The model under review builds one solid part; all positions refer to its coordinate system, in mm. A direction names the side the tool comes from. Coordinates: 2 decimals unless noted, no trailing zeros. Loops run counter-clockwise (first coordinate to the right, second up) from the corner with the lowest first, then second, coordinate; pieces in that order, holes last. Notation, with made-up numbers: (44, 87.25) - (57, 87.25) arc R35 cw to (57, 121.25) - close; hole circle Ø1 at (66.25, 66). An arc over 180 degrees is marked (long way). Answer in a Markdown table with one row per item. Add a question column.
(1) For P1, Ø5, axis at x = -135.5, z = 30, coming from the -Y side; P2, Ø4, axis at y = 152, z = 42.5, coming from the +X side; P3, Ø1, axis at x = -95, z = 32, coming from the +Y side, all flat-tipped, find the tip position at first contact; note any pin that passes through.
(2) For line 1 along Z through (x, y) = (-145.5, 86); line 2 along Y through (x, z) = (63.5, 31.5); line 3 along X through (y, z) = (0, 1), list the stretches that pass through material, from the lowest coordinate up.
(3) Mouldability with a two-part tool opening along Y and no side actions: class faces 3 (the cylindrical face through (-161.174, -35.79, 1.288)), 4 (the flat face through (-109, -124.5, 0)) as +Y half, -Y half, draft (parallel to the pull), parting line (faces both ways), or undercut.
(4) Machinability: for faces 1 (the flat face through (-95, 137, 2.54)), 2 (the flat face through (-109, 124.5, 50.8)), which of the approach directions +Z, -Z, +X, -X, +Y, -Y give a long, thin tool a straight path to every point of the face, cutting with its end or side? Answer none if there is none.
(5) We need section A-A on y = 0. Write out the cut boundary in (x, z).
(6) We need section C-C on z = 30.5. Write out the cut boundary in (x, y), plus the area to 3 significant figures.
from build123d import *


with BuildPart() as part:
    # Sketch1 → Revolve2 (revolve)
    with BuildSketch(Plane(origin=(0, 0, 0), x_dir=(0, 0, -1), z_dir=(1, 0, 0))):
        with BuildLine():
            Line((-50.8, 165.1), (-50.8, 185.42))
            ThreePointArc((-50.8, 185.42), (-25.4, 195.941024484), (0, 185.42))
            Line((0, 185.42), (0, 165.1))
            Line((0, 165.1), (-2.54, 165.1))
            Line((-2.54, 165.1), (-2.54, 184.345155613))
            ThreePointArc((-2.54, 184.345155613), (-25.4, 193.401024484), (-48.26, 184.345155613))
            Line((-48.26, 184.345155613), (-48.26, 165.1))
            Line((-48.26, 165.1), (-50.8, 165.1))
        make_face()
    revolve(axis=Axis((0, 0, 75.421455939), (0, 0, -1)))


solid = part.part
Outcome:
| question | item | result |
|---|---|---|
| 1 | P1 | y = -143.52 |
| 1 | P2 | x = 119.73 |
| 1 | P3 | y = 170.97 |
| 2 | line 1 | 0 to 2.54, 48.26 to 50.8 |
| 2 | line 2 | -184.81 to -182.08, 182.08 to 184.81 |
| 2 | line 3 | -186.38 to -165.1, 165.1 to 186.38 |
| 3 | face 3 | undercut |
| 3 | face 4 | draft |
| 4 | face 1 | none |
| 4 | face 2 | +Z, +X, -X, +Y, -Y |
| 5 | outline | (-185.42, 0) - (-165.1, 0) - (-165.1, 2.54) - (-184.35, 2.54) arc R33.38 cw to (-184.35, 48.26) - (-165.1, 48.26) - (-165.1, 50.8) - (-185.42, 50.8) arc R35.92 ccw to start; (165.1, 0) - (185.42, 0) arc R35.92 ccw to (185.42, 50.8) - (165.1, 50.8) - (165.1, 48.26) - (184.35, 48.26) arc R33.38 cw to (184.35, 2.54) - (165.1, 2.54) - close |
| 6 | outline | circle Ø391.15 at (0, 0); hole circle Ø386.02 at (0, 0) |
| 6 | area | 3,130 mm² |
